```python
from build123d import *

# Parameters (mm, degrees)
SKETCH_1_R           = 13.95
SKETCH_1_R_2         = 2.05
EXTRUDE_1_DEPTH      = 13.7
HOLE_WIZARD_M2_5_1_D = 2.05


with BuildPart() as part:
    # 草图1 → 凸台-拉伸1 (new body)
    with BuildSketch(Plane.XY):
        with Locations(Location((0, 0, 0), (0, 0, 180))):
            Circle(SKETCH_1_R)
        with Locations(Location((0, 0, 0), (0, 0, 180))):
            Circle(SKETCH_1_R_2, mode=Mode.SUBTRACT)
    extrude(amount=EXTRUDE_1_DEPTH)

    # M2.5 螺纹孔1 (through all)
    with Locations(Plane.XY.offset(13.7)):
        with Locations((0, 8.25), (8.25, 0), (0, -8.25), (-8.25, 0)):
            Hole(HOLE_WIZARD_M2_5_1_D / 2)


solid = part.part
```
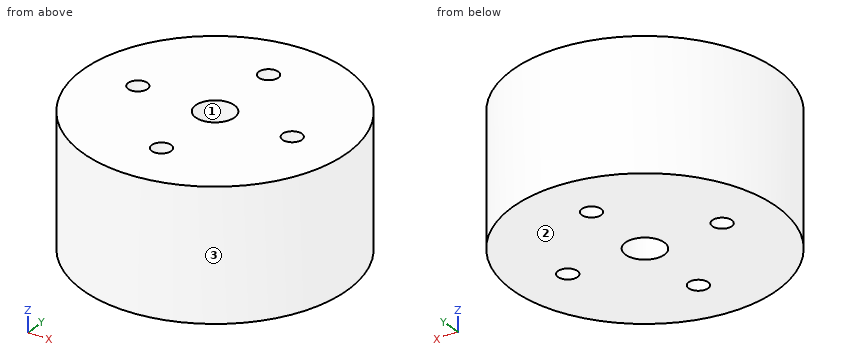
Build history of the part. All positions in model axes, mm. Face numbers are marked on the shaded views. Round coordinates to 2 decimals unless told otherwise and drop trailing zeros. Write each loop counter-clockwise with the first axis right and the second up, starting at its lowest first coordinate (ties: lowest second). Pieces come first, ordered by that corner, then holes. Notation, with made-up numbers: (7.25, 7) - (48.25, 7) arc R19 cw to (48.25, 33) - close; hole circle Ø1 at (86.5, 36). An arc over 180 degrees is marked (long way). Write each question's results on one line, items separated by ' | '. Start each with the question number.
Item 1: Drop flat-ended pins along their axis: P1, Ø5, axis at x = 5, z = 9, coming from the +Y side; P2, Ø5, axis at x = 10, z = 1.5, coming from the -Y side; P3, Ø2, axis at x = 9, z = 7, coming from the +Y side; P4, Ø3.5, axis at x = 0, y = 0, coming from the -Z side. Give the stop position or say it passes through.
Item 2: Mould opens along Y. For the marked faces 1, 2 and 3 say: pulls with the +Y half, pulls with the -Y half, needs draft (parallel to the pull), parting line crosses it, or undercut.
Item 3: Saw through at B-B (z = 5). Write the cut outline in (x, y) (3 decimals), and give its area (3 significant figures).
Item 4: Saw through at D-D (y = -5). Write the cut outline in (x, z).
Item 5: Saw through at C-C (x = -8.25). Write the cut outline in (y, z) (3 decimals).
Item 6: Wall check: L1, parallel to Y at x = 0, z = 10 (3 decimals); L2, parallel to X at y = -0.5, z = 3.75; L3, parallel to Y at x = -3.75, z = 4. Give the ranges that are in metal, low to high. Write a range as [from, to].
Item 7: Saw through at A-A (y = 1.5). Write the cut outline in (x, z).
Results are:
1) P1: stops at y = 13.72 | P2: stops at y = -11.76 | P3: stops at y = 11.43 | P4: passes through
2) face 1: undercut | face 2: needs draft | face 3: parting line crosses it
3) outline: circle Ø27.9 at (0, 0); hole circle Ø2.05 at (-8.25, 0); hole circle Ø4.1 at (0, 0); hole circle Ø2.05 at (0, -8.25); hole circle Ø2.05 at (0, 8.25); hole circle Ø2.05 at (8.25, 0) | area: 585 mm²
4) outline: (-13.02, 0) - (13.02, 0) - (13.02, 13.7) - (-13.02, 13.7) - close
5) outline: (-11.249, 0) - (-1.025, 0) - (-1.025, 13.7) - (-11.249, 13.7) - close; (1.025, 0) - (11.249, 0) - (11.249, 13.7) - (1.025, 13.7) - close
6) L1: y = [-13.95, -9.275], [-7.225, -2.05], [2.05, 7.225], [9.275, 13.95] | L2: x = [-13.94, -9.14], [-7.36, -1.99], [1.99, 7.36], [9.14, 13.94] | L3: y = [-13.44, 13.44]
7) outline: (-13.87, 0) - (-1.4, 0) - (-1.4, 13.7) - (-13.87, 13.7) - close; (1.4, 0) - (13.87, 0) - (13.87, 13.7) - (1.4, 13.7) - close
